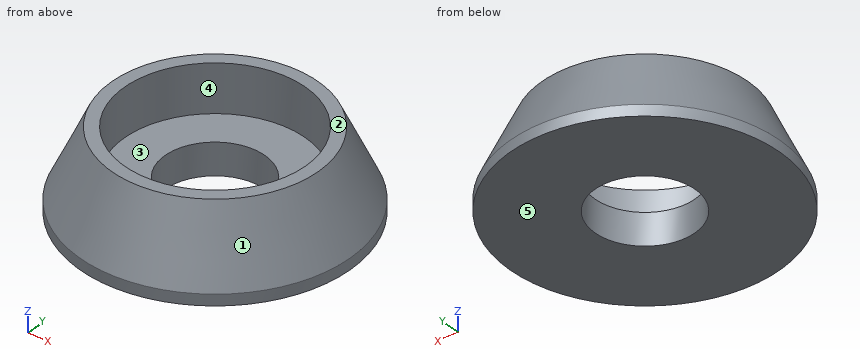
from build123d import *

# Parameters (mm, degrees)
F7_R  = 4.25
F8_R  = 4.25
F10_R = 3.25
F9_R  = 2.85
F11_R = 2.85
F13_R = 1.575
F12_R = 1.575


with BuildPart() as f14:
    # F7 (on Top) → F14 section 0
    with BuildSketch(Plane.XY):
        Circle(F7_R)
    # F8 (on offset) → F14 section 1
    with BuildSketch(Plane.XY.offset(0.35)):
        Circle(F8_R)
    loft()

    # F10 (on offset) → F15 section 0
    with BuildSketch(Plane.XY.offset(2.5)):
        Circle(F10_R)
    # F8 (on offset) → F15 section 1
    with BuildSketch(Plane.XY.offset(0.35)):
        Circle(F8_R)
    loft()

    # F9 (on offset) → F16 section 0
    with BuildSketch(Plane.XY.offset(2.5)):
        Circle(F9_R)
    # F11 (on offset) → F16 section 1
    with BuildSketch(Plane.XY.offset(1)):
        Circle(F11_R)
    loft(mode=Mode.SUBTRACT)

    # F13 (on offset) → F17 section 0
    with BuildSketch(Plane.XY.offset(1)):
        Circle(F13_R)
    # F12 (on Top) → F17 section 1
    with BuildSketch(Plane.XY):
        Circle(F12_R)
    loft(mode=Mode.SUBTRACT)


solid = f14.part
Here's how the part is built. I have some questions about the finished solid (model axes, mm). Face numbers are marked on the shaded views. A direction names the side the tool comes from. Give positions to 0.01 mm unless a question says otherwise; leave off trailing zeros. Order: outer loops, then holes, each group sorted by start corner. A loop starts at its lowest first (then second) coordinate and runs counter-clockwise, first axis right, second up. Notation, with made-up numbers: (56, 25) -> (108, 25) arc R12 ccw to (108, 43) -> close; hole circle Ø9 at (-36.75, -27). An arc over 180 degrees is marked (long way). Use a Markdown table: item, result. Add a question column.
Item 1: I need wall thicknesses on line 1 (Z direction, x = 1, y = -1.25); line 2 (Y direction, x = -2, z = 2.25); line 3 (Y direction, x = 0, z = 0.25) (3 decimals). Which ranges of each line are inside material? Lowest first, please.
Item 2: Imagine slicing it at A-A on x = 0. Please give me the cut outline in (y, z) (3 decimals), plus the area to 3 significant figures.
Item 3: For the marked faces 4 and 5, which set-ups out of +Z, -Z, +X, -X, +Y, -Y let a thin tool reach every point of the face, with its end or its side?
Item 4: If we mould it in two halves opening along Y, with no side actions, what happens to the marked faces 1, 2 and 3? For each: pulls with the +Y half, pulls with the -Y half, needs draft (parallel to the pull), parting line crosses it, or undercut.
Item 5: Imagine slicing it at B-B on z = 1.15. Please give me the cut outline in (x, y), plus the area to 3 significant figures.
Item 6: Will these pins go through, and if not, where does the flat tip stop? pin 1 (1.9 mm diameter, centred on x = 0, y = 0, fed in from -Z); pin 2 (1.5 mm diameter, centred on y = -2.5, z = 2, fed in from +X); pin 3 (1.7 mm diameter, centred on x = -1, y = 0.5, fed in from +Z); pin 4 (1 mm diameter, centred on x = -1.5, z = 2, fed in from -Y).
Item 7: Imagine slicing it at C-C on z = 0.5. Please give me the cut outline in (x, y) (3 decimals), plus the area to 3 significant figures.
Data:
| question | item | result |
|---|---|---|
| 1 | line 1 | z = 0 to 1 |
| 1 | line 2 | y = -2.71 to -2.03, 2.03 to 2.71 |
| 1 | line 3 | y = -4.25 to -1.575, 1.575 to 4.25 |
| 2 | outline | (-4.25, 0) -> (-1.575, 0) -> (-1.575, 1) -> (-2.85, 1) -> (-2.85, 2.5) -> (-3.25, 2.5) -> (-4.25, 0.35) -> close; (1.575, 0) -> (4.25, 0) -> (4.25, 0.35) -> (3.25, 2.5) -> (2.85, 2.5) -> (2.85, 1) -> (1.575, 1) -> close |
| 2 | area | 7.40 mm² |
| 3 | face 4 | +Z |
| 3 | face 5 | -Z, +X, -X, +Y, -Y |
| 4 | face 1 | parting line crosses it |
| 4 | face 2 | needs draft |
| 4 | face 3 | undercut |
| 5 | outline | circle Ø7.76 at (0, 0); hole circle Ø5.7 at (0, 0) |
| 5 | area | 21.7 mm² |
| 6 | pin 1 | passes through |
| 6 | pin 2 | stops at x = 3.17 |
| 6 | pin 3 | stops at z = 1 |
| 6 | pin 4 | stops at y = -3.47 |
| 7 | outline | circle Ø8.36 at (0, 0); hole circle Ø3.15 at (0, 0) |
| 7 | area | 47.1 mm² |
